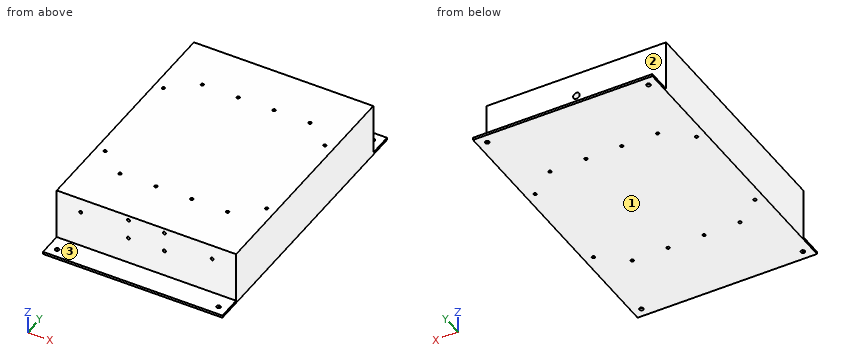
Autodesk Inventor part; units mm, degrees
ref_plane "YZ Plane" through (0, 0, 0) normal (1, 0, 0) x (0, 1, 0)
ref_plane "XZ Plane" through (0, 0, 0) normal (0, 1, 0) x (-1, 0, 0)
ref_plane "XY Plane" through (0, 0, 0) normal (0, 0, 1) x (1, 0, 0)
sketch "Sketch1" plane through (0, 0, 0) normal (0, 0, 1) x (1, 0, 0)
  line L0 (-75, -100) -> (75, -100)
  line L1 (75, -100) -> (75, 100)
  line L2 (75, 100) -> (-75, 100)
  line L3 (-75, 100) -> (-75, -100)
  line L4 (-75, -100) -> (75, 100) construction
  line L5 (75, -100) -> (-75, 100) construction
  point P0 (0, 0)
  dimension "d0" = 200
  dimension "d1" = 150
extrude "Extrusion1" add sketch "Sketch1" along normal blind 45
sketch "Sketch2" plane through (-75, 100, 0) normal (0, 1, 0) x (1, 0, 0)
  line L0 (150, 0) -> (150, -45)
  line L1 (0, 0) -> (150, 0)
  line L2 (150, 0) -> (150, -2)
  line L3 (150, -2) -> (0, -2)
  line L4 (0, -2) -> (0, 0)
  point P0 (75, 0)
  dimension "d4" = 2
extrude "Extrusion2" add sketch "Sketch2" along normal blind 20
sketch "Sketch3" plane through (-75, -100, 0) normal (0, -1, 0) x (1, 0, 0)
  line L0 (0, 0) -> (150, 0)
  line L1 (150, 0) -> (150, 45)
  line L2 (0, 0) -> (150, 0)
  line L3 (150, 0) -> (150, 2)
  line L4 (150, 2) -> (0, 2)
  line L5 (0, 2) -> (0, 0)
  point P0 (75, 0)
  dimension "d7" = 2
extrude "Extrusion3" add sketch "Sketch3" along normal blind 20
sketch "Sketch4" plane through (-75, -100, 2) normal (0, 0, 1) x (1, 0, 0)
  line L0 (7.5, 212.5) -> (142.5, 212.5) construction
  line L1 (142.5, 212.5) -> (142.5, -12.5) construction
  line L2 (142.5, -12.5) -> (7.5, -12.5) construction
  line L3 (7.5, -12.5) -> (7.5, 212.5) construction
  line L4 (0, 220) -> (150, 220)
  line L5 (150, -20) -> (0, -20) construction
  line L6 (0, 200) -> (0, 220) construction
  point P0 (75, 100)
  dimension "d10" = 135
  dimension "d11" = 7.5
  dimension "d12" = 7.5
  dimension "d13" = 150
  dimension "d14" = 7.5
  dimension "d34" = 225
hole "Hole1" at (-67.5, 112.5, 2) at (67.5, 112.5, 2) at (-67.5, -112.5, 2) at (67.5, -112.5, 2) direction (0, 0, -1) diameter 3.4 end through all
sketch "Sketch6" plane through (0, 0, 45) normal (0, 0, 1) x (1, 0, 0)
  line L0 (-67.5, 42.5) -> (67.5, 42.5) construction
  line L1 (67.5, 42.5) -> (67.5, -42.5) construction
  line L2 (67.5, -42.5) -> (-67.5, -42.5) construction
  line L3 (-67.5, -42.5) -> (-67.5, 42.5) construction
  line L4 (-67.5, 42.5) -> (67.5, -42.5) construction
  line L5 (67.5, 42.5) -> (-67.5, -42.5) construction
  line L6 (-45, 60) -> (45, 60) construction
  line L7 (45, 60) -> (45, -60) construction
  line L8 (45, -60) -> (-45, -60) construction
  line L9 (-45, -60) -> (-45, 60) construction
  line L10 (-45, 60) -> (45, -60) construction
  line L11 (45, 60) -> (-45, -60) construction
  line L12 (-15, -60) -> (15, -60) construction
  line L13 (15, -60) -> (15, 60) construction
  line L14 (15, 60) -> (-15, 60) construction
  line L15 (-15, 60) -> (-15, -60) construction
  line L16 (-15, -60) -> (15, 60) construction
  line L17 (15, -60) -> (-15, 60) construction
  point P0 (0, 0)
  dimension "d22" = 135
  dimension "d23" = 85
  dimension "d24" = 120
  dimension "d25" = 90
  dimension "d26" = 30
hole "Hole2" at (67.5, 42.5, 45) at (67.5, -42.5, 45) at (-67.5, -42.5, 45) at (-67.5, 42.5, 45) at (-45, -60, 45) at (-45, 60, 45) at (45, 60, 45) at (45, -60, 45) at (15, 60, 45) at (-15, 60, 45) at (-15, -60, 45) at (15, -60, 45) direction (0, 0, -1) diameter 2.459 end through all
sketch "Sketch9" plane through (-75, 100, 45) normal (0, 1, 0) x (1, 0, 0)
  line L0 (0, 43) -> (0, 0)
  line L1 (150, 0) -> (0, 0)
  point P0 (75, 45)
  point P1 (75, 20)
  dimension "d53" = 75
  dimension "d54" = 20
hole "Hole5" at (0, 100, 25) direction (0, -1, 0) diameter 5.5 depth 8 tip angle 118
sketch "Sketch11" plane through (-75, -100, 45) normal (0, -1, 0) x (1, 0, 0)
  line L0 (20, -20.5) -> (60, -20.5) construction
  line L1 (60, -20.5) -> (60, -4) construction
  line L2 (60, -4) -> (20, -4) construction
  line L3 (20, -4) -> (20, -20.5) construction
  line L4 (90, -20.5) -> (130, -20.5) construction
  line L5 (130, -20.5) -> (130, -4) construction
  line L6 (130, -4) -> (90, -4) construction
  line L7 (90, -4) -> (90, -20.5) construction
  line L8 (0, -45) -> (150, -45)
  line L9 (0, -43) -> (0, 0)
  point P0 (75, -45)
  point P1 (20, -12.25)
  point P2 (130, -12.25)
  dimension "d72" = 16.5
  dimension "d73" = 16.5
  dimension "d74" = 24.5
  dimension "d75" = 40
  dimension "d76" = 40
  dimension "d77" = 20
  dimension "d78" = 30
hole "Hole7" at (-15, -100, 41) at (-15, -100, 24.5) at (15, -100, 24.5) at (15, -100, 41) at (-55, -100, 32.75) at (55, -100, 32.75) direction (0, 1, 0) diameter 2.459 depth 10 tip angle 118
equation "\"d14\" = -0.5 * d10 + 0.5 * d13"
properties part number "Heatsink" material "Aluminum 6061"
Geometry: final body of the model. Coordinates: model frame, mm. Face numbers are marked on the shaded views. A direction names the side the tool comes from. Coordinates: 2 decimals unless noted, no trailing zeros. Write each loop counter-clockwise with the first axis right and the second up, starting at its lowest first coordinate (ties: lowest second). Pieces come first, ordered by that corner, then holes. Notation, with made-up numbers: M -6,-34.5 L 39,-34.5 A11 ccw 39,-24.5 Z; hole C 68.5,36 d8. An arc over 180 degrees is marked long. Use CSV: the item, a comma, the result in double quotes. Start each with the question number.
1. Cut plane B-B on x = -23. Return the cut outline in (y, z).
2. Ray query, probe 1 along Y at (x, z) = (-45, 9); probe 2 along X at (y, z) = (-112.5, 1.15); probe 3 along Y at (x, z) = (-67.5, 21.5). Return the intervals inside material, ascending.
3. Cut plane C-C on y = -103. Return the cut outline in (x, z).
4. First-contact query: P1, Ø8, axis at x = -21.5, z = 37, coming from the +Y side; P2, Ø3, axis at x = 15, y = -60, coming from the +Z side; P3, Ø4, axis at x = 67.5, y = 112.5, coming from the +Z side; P4, Ø2, axis at x = 15, z = 24.5, coming from the -Y side. Flat tips, straight axial feed; report the tip coordinate or a pass-through.
5. Reachability of the marked faces 1, 2 and 3 from +Z, -Z, +X, -X, +Y, -Y: full face, straight path, thin tool, end or side. Return the list, or none.
6. Cut plane A-A on z = 18. Count the separate pieces of the cut face and the enclosed holes in it, plus the area to 3 significant figures.
Entries:
1,outline,"M -120,0 L 120,0 L 120,2 L 100,2 L 100,45 L -100,45 L -100,2 L -120,2 Z"
2,probe 1,"-100 to -61.23, -58.77 to 58.77, 61.23 to 100"
2,probe 2,"-75 to -69.2, -65.8 to 65.8, 69.2 to 75"
2,probe 3,"-100 to -43.73, -41.27 to 41.27, 43.73 to 100"
3,outline,"M -75,0 L 75,0 L 75,2 L -75,2 Z"
4,P1,"y = 100"
4,P2,"z = 45"
4,P3,"z = 2"
4,P4,"y = -89.86"
5,face 1,"-Z, +X, -X, +Y, -Y"
5,face 2,"+Z, +X, -X, +Y"
5,face 3,"+Z, +X, -X, -Y"
6,separate pieces,"1"
6,enclosed holes,"12"
6,area,"29,900 mm²"
